Autodesk Inventor part; units mm, degrees
ref_plane "YZ Plane" through (0, 0, 0) normal (1, 0, 0) x (0, 1, 0)
ref_plane "XZ Plane" through (0, 0, 0) normal (0, 1, 0) x (-1, 0, 0)
ref_plane "XY Plane" through (0, 0, 0) normal (0, 0, 1) x (1, 0, 0)
sketch "スケッチ1" plane through (0, 0, 0) normal (0, 1, 0) x (-1, 0, 0)
  line L0 (0, 0) -> (-35, 0)
  line L1 (-35, 0) -> (-35, -220)
  line L2 (-35, -220) -> (0, -220)
  line L3 (0, -220) -> (0, 0)
  arc A0 (-35, -220) -> (0, -220) centre (-17.5, -220) ccw
  dimension "d0" = 35
  dimension "d1" = 220
  dimension "d2" = 17.5
extrude "押し出し1" add sketch "スケッチ1" along normal blind 3
sketch "スケッチ2" plane through (0, 3, 0) normal (0, 1, 0) x (1, 0, 0)
  line L0 (0, 0) -> (35, 0) construction
  line L1 (17.5, 0) -> (17.5, 237.5) construction
  arc A0 (35, 220) -> (0, 220) centre (17.5, 220) ccw construction
hole "穴1" at (17.5, 3, -220) direction (0, -1, 0) diameter 16 end through all
sketch "スケッチ3" plane through (0, 3, 0) normal (0, 1, 0) x (1, 0, 0)
  circle A0 centre (17.5, 220) radius 8
  circle A1 centre (17.5, 220) radius 12.5
  point P0 (0, 0)
  point P1 (5, 220)
  point P2 (30, 220)
  point P3 (17.5, 232.5)
  point P4 (17.5, 207.5)
  dimension "d12" = 25
hole "穴2" at (5, 3, -220) at (30, 3, -220) at (17.5, 3, -232.5) at (17.5, 3, -207.5) direction (0, -1, 0) diameter 2.459 end through all
sketch "スケッチ4" plane through (0, 3, 0) normal (0, 1, 0) x (1, 0, 0)
  line L0 (0, 0) -> (35, 0) construction
  line L1 (17.5, 0) -> (17.5, 237.5) construction
  arc A0 (35, 220) -> (0, 220) centre (17.5, 220) ccw construction
  circle A1 centre (17.5, 220) radius 8
  point P0 (17.5, 137)
  point P1 (17.5, 127)
  point P2 (17.5, 117)
  point P3 (17.5, 107)
  point P4 (17.5, 97)
  point P5 (17.5, 87)
  point P6 (17.5, 77)
  point P7 (17.5, 67)
  point P8 (17.5, 57)
  point P9 (17.5, 47)
  point P10 (17.5, 37)
  point P11 (17.5, 27)
  point P12 (17.5, 17)
  point P13 (17.5, 7)
  dimension "d42" = 83
  dimension "d45" = 10
hole "穴3" at (17.5, 3, -137) at (17.5, 3, -127) at (17.5, 3, -117) at (17.5, 3, -107) at (17.5, 3, -97) at (17.5, 3, -87) at (17.5, 3, -77) at (17.5, 3, -67) at (17.5, 3, -57) at (17.5, 3, -47) at (17.5, 3, -37) at (17.5, 3, -27) at (17.5, 3, -17) at (17.5, 3, -7) direction (0, -1, 0) diameter 3.2 end through all
sketch "スケッチ5" plane through (0, 3, 0) normal (0, 1, 0) x (1, 0, 0)
  line L0 (0, 0) -> (35, 0) construction
  line L1 (17.5, 0) -> (17.5, 237.5) construction
  arc A0 (35, 220) -> (0, 220) centre (17.5, 220) ccw construction
  circle A1 centre (17.5, 137) radius 1.6 construction
  point P0 (17.5, 150)
  point P1 (17.5, 170)
  dimension "d50" = 13
  dimension "d51" = 20
hole "穴4" at (17.5, 3, -150) at (17.5, 3, -170) direction (0, -1, 0) diameter 6.6 end through all
properties part number "shoulder2_upper_plate_left" material "アルミニウム 5052"
Can you work these out from the model? Positions are in its coordinate system, mm. Give positions to 0.01 mm unless a question says otherwise; leave off trailing zeros. Use a Markdown table: item, result. Add a question column.
Q1. Please list where these lines run through material, in increasing order: line 1 along X through (y, z) = (1.3, -220); line 2 along X through (y, z) = (2.65, -56); line 3 along X through (y, z) = (2.75, -27).
Q2. If we section it at A-A on y = 1: Count the separate pieces of the cut face and the enclosed holes in it, plus the area to 3 significant figures.
Q3. If we mould it in two halves opening along Z, with no side actions, what happens to faces 1 (the cylindrical face through (15.27, 1.48, -152.43)), 2 (the flat face through (22, 3, -117)), 3 (the cylindrical face through (17.115, 1.479, -237.496))? For each: released by +Z, released by -Z, zero draft, split by the parting line, or undercut.
Answers follow:
| question | item | result |
|---|---|---|
| 1 | line 1 | x = 0 to 3.77, 6.23 to 9.5, 25.5 to 28.77, 31.23 to 35 |
| 1 | line 2 | x = 0 to 16.25, 18.75 to 35 |
| 1 | line 3 | x = 0 to 15.9, 19.1 to 35 |
| 2 | separate pieces | 1 |
| 2 | enclosed holes | 21 |
| 2 | area | 7,780 mm^2 |
| 3 | face 1 | undercut |
| 3 | face 2 | zero draft |
| 3 | face 3 | released by -Z |
